Here's how the part is built. I have some questions about the finished solid (model axes, mm). A direction names the side the tool comes from. Coordinates: 2 decimals unless noted, no trailing zeros. Loops run counter-clockwise (first coordinate to the right, second up) from the corner with the lowest first, then second, coordinate; pieces in that order, holes last. Notation, with made-up numbers: (60.5, -17) - (116.5, -17) arc R16 ccw to (116.5, 7) - close; hole circle Ø10 at (17, -14.5). An arc over 180 degrees is marked (long way). Use a Markdown table: item, result.
```python
from build123d import *
from build123d.topology import SkipClean

# Parameters (mm, degrees)
SKETCH1_R                 = 8.5
BASE_EXTRUDE_DEPTH        = 110
SKETCH1_4_R               = 22.5
FRONT_CAP_DEPTH           = 4.5
END_BEVEL_FILLET_R        = 1
SKETCH7_R                 = 8.5
FRONT_KNOB_DEPTH          = 4
FRONT_KNOB_SLOT_DEPTH     = 23
M7X1_0_TAPPED_HOLE1_D     = 6
M7X1_0_TAPPED_HOLE1_DEPTH = 19
M7X1_0_TAPPED_HOLE1_TIP   = 1.802581857


with BuildPart() as part:
    # Sketch1 → Base Extrude (new body)
    with BuildSketch(Plane.XY):
        Circle(SKETCH1_R)
    extrude(amount=-BASE_EXTRUDE_DEPTH)

    # Sketch1_4 → Front Cap (add, symmetric)
    with BuildSketch(Plane.XY):
        Circle(SKETCH1_4_R)
    extrude(amount=FRONT_CAP_DEPTH, both=True)

    # Sketch3 → End Bevel (revolve, cut)
    with BuildSketch(Plane(origin=(0, 0, 0), x_dir=(0, 0, -1), z_dir=(1, 0, 0)), mode=Mode.PRIVATE) as end_bevel_sk:
        Polygon((74.010644069, 8.5), (114, 0), (124.010644069, 0), (124.010644069, 25), (74.010644069, 25), align=None)
    revolve(end_bevel_sk.sketch.rotate(Axis((0, 0, -92.509493434), (0, 0, -1)), 90), axis=Axis((0, 0, -92.509493434), (0, 0, -1)), mode=Mode.SUBTRACT)  # turned: the seam where the file's is

    # End Bevel Fillet
    end_bevel_fillet_edges = [part.edges().sort_by_distance(p)[0] for p in [
        (-0.850226247, 0, -110),
    ]]
    fillet(end_bevel_fillet_edges, radius=END_BEVEL_FILLET_R)

    # Sketch7 → Front Knob (add)
    with BuildSketch(Plane.XY.offset(4.5)):
        Circle(SKETCH7_R)
    extrude(amount=FRONT_KNOB_DEPTH)

    # Sketch6 → Front Knob Slot (add)
    with SkipClean():  # keep this step's faces unmerged: merging them makes the solid invalid here
        with BuildSketch(Plane.XY.offset(8.5)):
            with BuildLine():
                Line((-4.25, -7.361215932), (-4.25, 7.361215932))
                ThreePointArc((-4.25, 7.361215932), (0, 8.5), (4.25, 7.361215932))
                Line((4.25, 7.361215932), (4.25, -7.361215932))
                ThreePointArc((4.25, -7.361215932), (0, -8.5), (-4.25, -7.361215932))
            make_face()
        extrude(amount=FRONT_KNOB_SLOT_DEPTH)

    # M7x1.0 Tapped Hole1
    with Locations(Plane.XY.offset(31.5)):
        with Locations((0, 0)):
            Hole(M7X1_0_TAPPED_HOLE1_D / 2, depth=M7X1_0_TAPPED_HOLE1_DEPTH)
            with Locations((0, 0, -(M7X1_0_TAPPED_HOLE1_DEPTH + M7X1_0_TAPPED_HOLE1_TIP / 2))):  # 118° drill point
                Cone(0, M7X1_0_TAPPED_HOLE1_D / 2, M7X1_0_TAPPED_HOLE1_TIP, mode=Mode.SUBTRACT)


solid = part.part
```
Q1. I want a section at C-C, the plane x = -17.5. Write out the boundary of the cut face in (y, z).
Check values:
| item | result |
|---|---|
| outline | (-14.14, -4.5) - (14.14, -4.5) - (14.14, 4.5) - (-14.14, 4.5) - close |
Q2. If we mould it in two halves opening along X, with no side actions, what happens to faces 1 (the face through (3, 0, 22)), 2 (the face through (3, -2, 31.5)), 3 (the face through (4.57, 7.167, -38.769))? For each: pulls with the +X half, pulls with the -X half, needs draft (parallel to the pull), parting line crosses it, or undercut.
Check values:
| item | result |
|---|---|
| face 1 | undercut |
| face 2 | needs draft |
| face 3 | parting line crosses it |
Q3. I want a section at A-A, the plane z = -71.5. Write out the boundary of the cut face in (x, y), then the cut area to 3 significant figures.
Check values:
| item | result |
|---|---|
| outline | circle Ø17 at (0, 0) |
| area | 227 mm^2 |
Q4. I want a section at B-B, the plane y = 15.5. Write out the boundary of the cut face in (x, z), then the cut area to 3 significant figures.
Check values:
| item | result |
|---|---|
| outline | (-16.31, -4.5) - (16.31, -4.5) - (16.31, 4.5) - (-16.31, 4.5) - close |
| area | 294 mm^2 |
Q5. Please list where these lines run through material, in increasing order: L1, parallel to X at y = 0, z = 27; L2, parallel to Y at x = 0, z = 22.5; L3, parallel to Z at x = -6.5, y = -12. Write a range as from..to.
Check values:
| item | result |
|---|---|
| L1 | -4.25..-3, 3..4.25 |
| L2 | -8.5..-3, 3..8.5 |
| L3 | -4.5..4.5 |
Q6. Which directions (+Z, -Z, +X, -X, +Y, -Y) give clear straight access to the entire face, cutting with the end or side of a thin tool? Please do faces 4 (the face through (10, 0, 4.5)), 5 (the face through (6, 0, 8.5)), 6 (the face through (-4.25, 0, 20)).
Check values:
| item | result |
|---|---|
| face 4 | +Z |
| face 5 | +Z, +X, +Y, -Y |
| face 6 | +Z, -X, +Y, -Y |
Q7. I want a section at D-D, the plane z = -88. Write out the boundary of the cut face in (x, y).
Check values:
| item | result |
|---|---|
| outline | circle Ø11.05 at (0, 0) |
Q8. Will these pins go through, and if not, where does the flat tip stop? P1, Ø7.5, axis at y = -0.5, z = 19.5, coming from the -X side; P2, Ø6, axis at x = -12.5, z = -50.5, coming from the +Y side; P3, Ø2, axis at y = 7, z = -42, coming from the +X side; P4, Ø4, axis at x = -7.5, y = 1.5, coming from the +Z side.
Check values:
| item | result |
|---|---|
| P1 | x = -4.25 |
| P2 | through |
| P3 | x = 6.02 |
| P4 | z = 8.5 |
